```python
from build123d import *

# Parameters (mm, degrees)
F0_R     = 3.175
F0_R_2   = 1.5875
F1_DEPTH = 25.4


with BuildPart() as f1:
    # F0 (on Front) → F1 (new body)
    with BuildSketch(Plane.XZ):
        with BuildLine():
            ThreePointArc((-9.5081937086, 58.0158391523), (-0.2829133485, 47.9294646022), (9.525, 57.4502621022))
            ThreePointArc((9.525, 57.4502621022), (0.2829133485, 66.9710596023), (-9.5081937086, 58.0158391523))
        make_face()
        with Locations((0, 57.4502621022)):
            Circle(F0_R, mode=Mode.SUBTRACT)
        with BuildLine():
            Line((15.3865384615, 10.5579544099), (9.525, 57.4502621022))
            ThreePointArc((9.525, 57.4502621022), (-0.2829133485, 47.9294646022), (-9.5081937086, 58.0158391523))
            Line((-9.5081937086, 58.0158391523), (-15.393400304, 10.5308357814))
            ThreePointArc((-15.393400304, 10.5308357814), (-0.0139866445, 22.5252559408), (15.3865384615, 10.5579544099))
        make_face()
        with Locations((-3.1419943552, 43.1754621022)):
            Circle(F0_R_2, mode=Mode.SUBTRACT)
        with BuildLine():
            Line((15.875, 6.6502621022), (15.3865384615, 10.5579544099))
            ThreePointArc((15.3865384615, 10.5579544099), (-0.0139866445, 22.5252559408), (-15.393400304, 10.5308357814))
            Line((-15.393400304, 10.5308357814), (-15.8749991405, 6.6450380613))
            Line((-15.8749991405, 6.6450380613), (-15.5661926872, 3.5342919124))
            ThreePointArc((-15.5661926872, 3.5342919124), (-0.002485721, -9.2247377032), (15.5652161214, 3.5294173299))
            Line((15.5652161214, 3.5294173299), (15.875, 6.6502621022))
        make_face()
        with Locations((0, 6.6502621022)):
            Circle(F0_R, mode=Mode.SUBTRACT)
        with BuildLine():
            ThreePointArc((15.875, 6.6502621022), (15.7524112928, 8.6193135138), (15.3865384615, 10.5579544099))
            Line((15.3865384615, 10.5579544099), (15.875, 6.6502621022))
        make_face()
        with BuildLine():
            Line((-15.8749991405, 6.6450380613), (-15.393400304, 10.5308357814))
            ThreePointArc((-15.393400304, 10.5308357814), (-15.754461493, 8.6028419507), (-15.8749991405, 6.6450380613))
        make_face()
        with BuildLine():
            ThreePointArc((15.5652161214, 3.5294173299), (15.7973641936, 5.0821710538), (15.875, 6.6502621022))
            Line((15.875, 6.6502621022), (15.5652161214, 3.5294173299))
        make_face()
        with BuildLine():
            Line((-15.5661926872, 3.5342919124), (-15.8749991405, 6.6450380613))
            ThreePointArc((-15.8749991405, 6.6450380613), (-15.7973517175, 5.0820453721), (-15.5661926872, 3.5342919124))
        make_face()
        with BuildLine():
            Line((11.1487181344, -40.9635521522), (15.5652161214, 3.5294173299))
            ThreePointArc((15.5652161214, 3.5294173299), (-0.002485721, -9.2247377032), (-15.5661926872, 3.5342919124))
            Line((-15.5661926872, 3.5342919124), (-9.4784110305, -57.7906679359))
            ThreePointArc((-9.4784110305, -57.7906679359), (-0.4710413646, -47.33639227), (9.525, -56.8497378978))
            ThreePointArc((9.525, -56.8497378978), (6.9705567315, -63.341036986), (0.6773435479, -66.3506236838))
            Line((0.6773435479, -66.3506236838), (44.7324052746, -64.7822125124))
            ThreePointArc((44.7324052746, -64.7822125124), (36.5137564458, -56.9909628899), (44.45, -48.9122378978))
            Line((44.45, -48.9122378978), (17.2401500444, -47.9367114742))
            ThreePointArc((17.2401500444, -47.9367114742), (12.6853766448, -45.7683751299), (11.1487181344, -40.9635521522))
        make_face()
        with BuildLine():
            ThreePointArc((9.525, -56.8497378978), (-0.4710413646, -47.33639227), (-9.4784110305, -57.7906679359))
            ThreePointArc((-9.4784110305, -57.7906679359), (-6.393874662, -63.9097656461), (0, -66.3747378978))
            Line((0, -66.3747378978), (0.6773435479, -66.3506236838))
            ThreePointArc((0.6773435479, -66.3506236838), (6.9705567315, -63.341036986), (9.525, -56.8497378978))
        make_face()
        with Locations((0, -56.8497378978)):
            Circle(F0_R, mode=Mode.SUBTRACT)
        with BuildLine():
            Line((0.6773435479, -66.3506236838), (0, -66.3747378978))
            ThreePointArc((0, -66.3747378978), (0.3388863295, -66.3687074353), (0.6773435479, -66.3506236838))
        make_face()
        with BuildLine():
            ThreePointArc((52.3875, -56.8497378978), (50.0626600757, -51.2370778221), (44.45, -48.9122378978))
            ThreePointArc((44.45, -48.9122378978), (36.5137564458, -56.9909628899), (44.7324052746, -64.7822125124))
            ThreePointArc((44.7324052746, -64.7822125124), (50.1616327839, -62.3616483825), (52.3875, -56.8497378978))
        make_face()
        with Locations((44.45, -56.8497378978)):
            Circle(F0_R, mode=Mode.SUBTRACT)
    extrude(amount=F1_DEPTH)


solid = f1.part
```
The listing builds one solid part. Answer for the finished solid, in the listing's coordinates (mm). A direction names the side the tool comes from. Round coordinates to 2 decimals unless told otherwise and drop trailing zeros. Order: outer loops, then holes, each group sorted by start corner. A loop starts at its lowest first (then second) coordinate and runs counter-clockwise, first axis right, second up. Notation, with made-up numbers: (52, 19) -> (82, 19) arc R23 ccw to (82, 49) -> close; hole circle Ø4 at (-23, 55.5). An arc over 180 degrees is marked (long way). Answer as CSV lines item,"result".
Q1. Consider line 1 (Z direction, x = 0, y = -6.25); line 2 (X direction, y = -14.5, z = -58); line 3 (Z direction, x = 2, y = -13.5). Determine where each line is inside the solid, lowest interval first. Write a range as from..to.
Computed values:
line 1,"z = -66.37..-60.02, -53.67..3.48, 9.83..54.28, 60.63..66.98"
line 2,"x = -9.46..-2.96, 2.96..41.49, 47.41..52.3"
line 3,"z = -66.3..-59.32, -54.38..4.18, 9.12..54.98, 59.92..66.76"
Q2. A cutting plane is placed at B-B on z = 53. Determine the outline of the cut face in (x, y).
Computed values:
outline,"(-10.13, -25.4) -> (10.08, -25.4) -> (10.08, 0) -> (-10.13, 0) -> close"
Q3. A cutting plane is placed at C-C on x = -8. Determine the outline of the cut face in (y, z), plus the area to 3 significant figures.
Computed values:
outline,"(-25.4, -62.02) -> (0, -62.02) -> (0, 62.62) -> (-25.4, 62.62) -> close"
area,"3,170 mm^2"
Q4. Given pin 1 (3 mm diameter, centred on x = 23, y = -3, fed in from +Z); pin 2 (1 mm diameter, centred on x = -3.5, y = -12, fed in from +Z); pin 3 (3 mm diameter, centred on x = 34.5, y = -7.5, fed in from +Z), each flat-ended and moving along its own axis, determine where each tip first touches the part or whether it passes through.
Computed values:
pin 1,"stops at z = -48.09"
pin 2,"stops at z = 66.49"
pin 3,"stops at z = -48.5"
Q5. Which of the six approach directions +Z, -Z, +X, -X, +Y, -Y give full straight-line access (tool end or side, diameter ignored) to faces 1 (the flat face through (13.326, -12.522, -19.029)), 2 (the cylindrical face through (0.488, -12.522, 66.963))?
Computed values:
face 1,"+X, +Y, -Y"
face 2,"+Z, +Y, -Y"
Q6. A cutting plane is placed at A-A on y = -16.25. Give the number of separate pieces and of enclosed holes in the cut face, plus the area to 3 significant figures.
Computed values:
separate pieces,"1"
enclosed holes,"5"
area,"3,780 mm^2"
